Work out the finished part from the listing and answer in its coordinate system (mm). Face numbers are marked on the shaded views. A direction names the side the tool comes from. Round coordinates to 2 decimals unless told otherwise and drop trailing zeros. Loops run counter-clockwise (first coordinate to the right, second up) from the corner with the lowest first, then second, coordinate; pieces in that order, holes last. Notation, with made-up numbers: M 31,17 L 81,17 A11 ccw 81,27 Z; hole C -8,23.25 d3. An arc over 180 degrees is marked long. One line per item, written item: value.
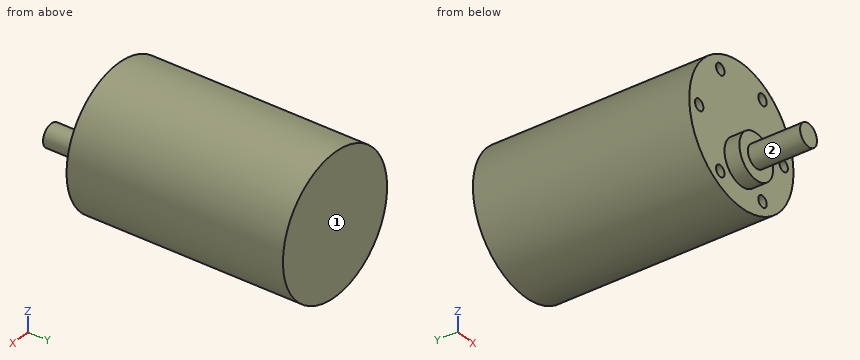
```python
from build123d import *

# Parameters (mm, degrees)
F0_R     = 18.5
F0_R_2   = 1.5
F0_R_3   = 6
F0_R_4   = 3
F1_DEPTH = 58
F2_DEPTH = 4
F3_DEPTH = 18
F4_DEPTH = 25


with BuildPart() as f1:
    # F0 (on Front) → F1 (new body)
    with BuildSketch(Plane.XZ):
        Circle(F0_R)
        with Locations((-7.5, -12.990381)):
            Circle(F0_R_2, mode=Mode.SUBTRACT)
        with Locations((7.5, -12.990381)):
            Circle(F0_R_2, mode=Mode.SUBTRACT)
        with Locations((0, -7)):
            Circle(F0_R_3, mode=Mode.SUBTRACT)
        with Locations((-15, 0)):
            Circle(F0_R_2, mode=Mode.SUBTRACT)
        with Locations((-7.5, 12.990381)):
            Circle(F0_R_2, mode=Mode.SUBTRACT)
        with Locations((15, 0)):
            Circle(F0_R_2, mode=Mode.SUBTRACT)
        with Locations((7.5, 12.990381)):
            Circle(F0_R_2, mode=Mode.SUBTRACT)
        with Locations((0, -7)):
            Circle(F0_R_3)
        with Locations((0, -7)):
            Circle(F0_R_4, mode=Mode.SUBTRACT)
        with Locations((0, -7)):
            Circle(F0_R_4)
        with Locations((-7.5, 12.990381)):
            Circle(F0_R_2)
        with Locations((7.5, 12.990381)):
            Circle(F0_R_2)
        with Locations((15, 0)):
            Circle(F0_R_2)
        with Locations((7.5, -12.990381)):
            Circle(F0_R_2)
        with Locations((-7.5, -12.990381)):
            Circle(F0_R_2)
        with Locations((-15, 0)):
            Circle(F0_R_2)
    extrude(amount=-F1_DEPTH)

    # F0 (on Front) → F2 (join)
    with BuildSketch(Plane.XZ):
        with Locations((0, -7)):
            Circle(F0_R_3)
        with Locations((0, -7)):
            Circle(F0_R_4, mode=Mode.SUBTRACT)
        with Locations((0, -7)):
            Circle(F0_R_4)
    extrude(amount=F2_DEPTH)

    # F0 (on Front) → F3 (join)
    with BuildSketch(Plane.XZ):
        with Locations((0, -7)):
            Circle(F0_R_4)
    extrude(amount=F3_DEPTH)

    # F0 (on Front) → F4 (cut)
    with BuildSketch(Plane.XZ):
        with Locations((7.5, 12.990381)):
            Circle(F0_R_2)
        with Locations((-7.5, 12.990381)):
            Circle(F0_R_2)
        with Locations((-15, 0)):
            Circle(F0_R_2)
        with Locations((7.5, -12.990381)):
            Circle(F0_R_2)
        with Locations((15, 0)):
            Circle(F0_R_2)
        with Locations((-7.5, -12.990381)):
            Circle(F0_R_2)
    extrude(amount=-F4_DEPTH, mode=Mode.SUBTRACT)


solid = f1.part
```
1) For the marked faces 1 and 2, determine the directions among +Z, -Z, +X, -X, +Y, -Y from which every point of the face is accessible in a straight line to the end or side of a thin tool.
Check values:
face 1: +Z, -Z, +X, -X, +Y
face 2: -Y
2) Find section B-B (x = 0). Give the vertices of the cut face in (y, z), then the cut area to 3 significant figures.
Check values:
outline: M -18,-10 L -4,-10 L -4,-13 L 0,-13 L 0,-18.5 L 58,-18.5 L 58,18.5 L 0,18.5 L 0,-1 L -4,-1 L -4,-4 L -18,-4 Z
area: 2,280 mm2
3) Find the intervals of material crossed by probe 1 along Y at (x, z) = (15, 3.5); probe 2 along Z at (x, y) = (-7, 14); probe 3 along Y at (x, z) = (5.5, -5), in increasing order. Write a range as from..to.
Check values:
probe 1: 0..58
probe 2: -17.12..-14.4, -11.58..11.58, 14.4..17.12
probe 3: -4..58
4) Find section D-D (x = 15). Give the vertices of the cut face in (y, z).
Check values:
outline: M 0,-10.83 L 58,-10.83 L 58,10.83 L 0,10.83 L 0,1.5 L 25,1.5 L 25,-1.5 L 0,-1.5 Z
5) Find section A-A (z = 0). Give the vertices of the cut face in (x, y).
Check values:
outline: M -18.5,0 L -16.5,0 L -16.5,25 L -13.5,25 L -13.5,0 L 13.5,0 L 13.5,25 L 16.5,25 L 16.5,0 L 18.5,0 L 18.5,58 L -18.5,58 Z
6) Find section C-C (y = 15). Give the vertices of the cut face in (x, z), then the cut area to 3 significant figures.
Check values:
outline: C 0,0 d37; hole C -15,0 d3; hole C -7.5,-12.99 d3; hole C -7.5,12.99 d3; hole C 7.5,-12.99 d3; hole C 7.5,12.99 d3; hole C 15,0 d3
area: 1,030 mm2
7) Each of these flat-tipped pins is pushed along its axis until it touches: pin 1 (4 mm diameter, centred on x = -0.5, y = 46.5, fed in from -Z); pin 2 (0.9 mm diameter, centred on x = 8, z = 12.5, fed in from -Y); pin 3 (3 mm diameter, centred on y = 33, z = -2.5, fed in from -X). Where does it stop, or does it pass through?
Check values:
pin 1: z = -18.5
pin 2: y = 25
pin 3: x = -18.47
